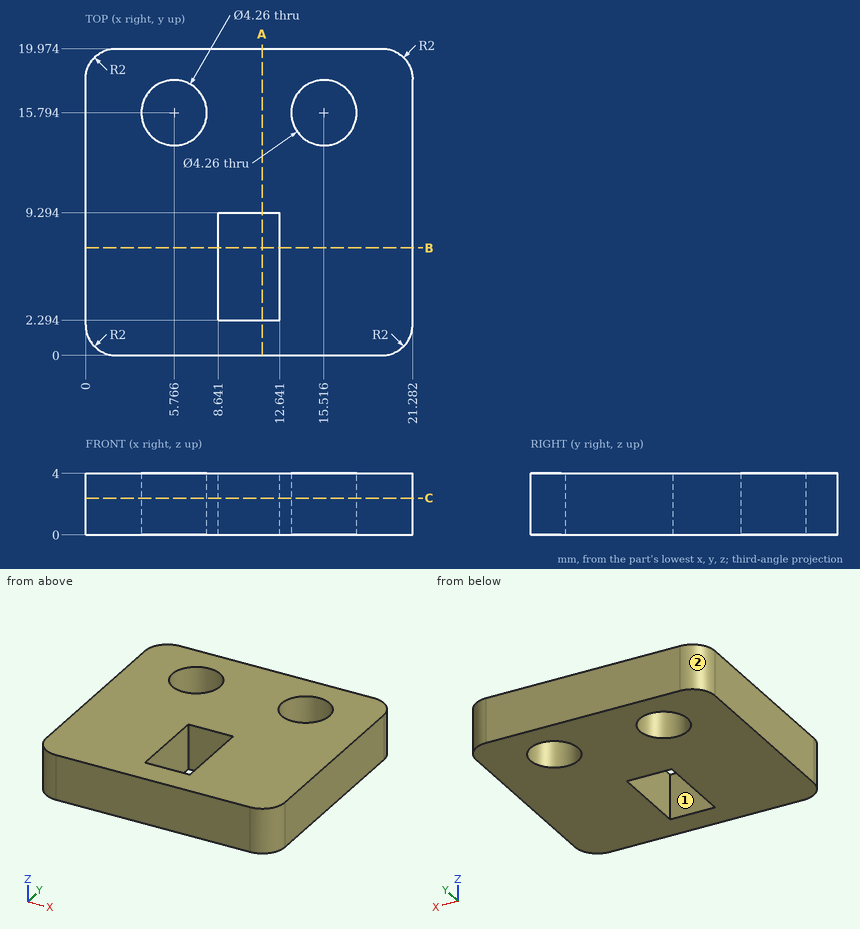
Check sheet for the drawn part. Datum: minimum x, y, z corner. Units: mm. A direction names the side the tool comes from. Give positions to 0.01 mm unless a question says otherwise; leave off trailing zeros. Write each loop counter-clockwise with the first axis right and the second up, starting at its lowest first coordinate (ties: lowest second). Pieces come first, ordered by that corner, then holes. Notation, with made-up numbers: M 44.25,78.5 L 74.25,78.5 A13 cw 74.25,87.5 Z; hole C 43.5,61.25 d2. An arc over 180 degrees is marked long. One line per question, with ' | ' between items.
1) Section check B-B on y = 7. Enter the section's corners in (x, z), plus the area to 3 significant figures.
Result:
outline: M 0,0 L 8.64,0 L 8.64,4 L 0,4 Z; M 12.64,0 L 21.28,0 L 21.28,4 L 12.64,4 Z | area: 69.1 mm2
2) Thickness scan on line 1 along X through (y, z) = (8.75, 0.2); line 2 along Y through (x, z) = (12.5, 2); line 3 along X through (y, z) = (17.5, 1.45). Record the ranges inside material, lowest first. Write a range as [from, to].
Result:
line 1: x = [0, 8.64], [12.64, 21.28] | line 2: y = [0, 2.29], [9.29, 19.97] | line 3: x = [0, 4.49], [7.04, 14.24], [16.79, 21.28]
3) Section check A-A on x = 11.5. Enter the section's corners in (y, z), plus the area to 3 significant figures.
Result:
outline: M 0,0 L 2.29,0 L 2.29,4 L 0,4 Z; M 9.29,0 L 19.97,0 L 19.97,4 L 9.29,4 Z | area: 51.9 mm2
4) Set-up check for the marked faces 1 and 2: record each of +Z, -Z, +X, -X, +Y, -Y from which the full face is reachable in a straight line by a thin tool's end or side.
Result:
face 1: +Z, -Z | face 2: +Z, -Z, -X, +Y
5) Section check C-C on z = 2.4. Enter the section's corners in (x, y).
Result:
outline: M 0,2 A2 ccw 2,0 L 19.28,0 A2 ccw 21.28,2 L 21.28,17.97 A2 ccw 19.28,19.97 L 2,19.97 A2 ccw 0,17.97 Z; hole C 5.77,15.79 d4.26; hole M 8.64,2.29 L 12.64,2.29 L 12.64,9.29 L 8.64,9.29 Z; hole C 15.52,15.79 d4.26
